Check sheet for the modelled part. Datum: model origin and axes. Units: mm. A direction names the side the tool comes from. Round coordinates to 2 decimals unless told otherwise and drop trailing zeros. Write each loop counter-clockwise with the first axis right and the second up, starting at its lowest first coordinate (ties: lowest second). Pieces come first, ordered by that corner, then holes. Notation, with made-up numbers: (20, 79.5) - (32, 79.5) arc R12 ccw to (32, 92.5) - close; hole circle Ø2 at (-11, -18). An arc over 180 degrees is marked (long way). Use one line per item in the form item = value. Start each with the question number.
1) Section check B-B (y = 20.5). Count the separate pieces of the cut face and the enclosed holes in it, then the cut area to 3 significant figures.
2) Section check D-D (z = 21). Record the boundary of the cut face in (x, y), then the cut area to 3 significant figures.
3) Set-up check for faces 1 (the face through (-13, -25.4, 7)), 2 (the face through (16, 0, -4.762)): record each of +Z, -Z, +X, -X, +Y, -Y from which the full face is reachable in a straight line by a thin tool's end or side.
4) Section check C-C (x = 65). Record the boundary of the cut face in (y, z).
5) Gauge pin test, flat ends, axial feed: P1, Ø3, axis at x = -14.5, y = 7.5, coming from the -Z side; P2, Ø2, axis at y = 20, z = -2, coming from the +X side; P3, Ø6, axis at x = -17, y = 4, coming from the +Z side. Record the tip position at first contact, or that the pin passes through.
6) Draft check along Z on faces 3 (the face through (22, 25.4, 0)), 4 (the face through (30.824, 12.522, -23.504)), 5 (the face through (0.246, 0.356, -14.285)). Enter one of: +Z half, -Z half, draft (parallel to the pull), parting line (faces both ways), or undercut.
7) Section check A-A (x = 0). Record the boundary of the cut face in (y, z) (1 decimal), then the cut area to 3 significant figures.
8) Scan lines: probe 1 along X at (y, z) = (22.5, -0.5); probe 2 along X at (y, z) = (7, 11); probe 3 along Y at (x, z) = (35, 19.5). Record each from-to range of solid material in increasing order.
from build123d import *

# Parameters (mm, degrees)
F0_R     = 14.2875
F1_DEPTH = 25.4
F2_DEPTH = 25.4


with BuildPart() as f1:
    # F0 (on Front) → F1 (new body)
    with BuildSketch(Plane.XZ):
        with BuildLine():
            ThreePointArc((5.042647, -28.126541), (21.916025, -18.336262), (28.575, 0))
            ThreePointArc((28.575, 0), (21.916025, 18.336262), (5.042647, 28.126541))
            ThreePointArc((5.042647, 28.126541), (-28.575, 0), (5.042647, -28.126541))
        make_face()
        with BuildLine():
            ThreePointArc((-13.470384, 4.7625), (0, 14.2875), (13.470384, 4.7625))
            Line((13.470384, 4.7625), (19.05, 4.7625))
            Line((19.05, 4.7625), (19.05, -4.7625))
            Line((19.05, -4.7625), (13.470384, -4.7625))
            ThreePointArc((13.470384, -4.7625), (0, -14.2875), (-13.470384, -4.7625))
            Line((-13.470384, -4.7625), (-19.05, -4.7625))
            Line((-19.05, -4.7625), (-19.05, 4.7625))
            Line((-19.05, 4.7625), (-13.470384, 4.7625))
        make_face(mode=Mode.SUBTRACT)
        with BuildLine():
            ThreePointArc((73.025, 0), (68.585683, 12.224174), (57.336765, 18.751028))
            ThreePointArc((57.336765, 18.751028), (34.925, 0), (57.336765, -18.751028))
            ThreePointArc((57.336765, -18.751028), (68.585683, -12.224174), (73.025, 0))
        make_face()
        with Locations((53.975, 0)):
            Circle(F0_R, mode=Mode.SUBTRACT)
        with BuildLine():
            ThreePointArc((5.042647, 28.126541), (21.916025, 18.336262), (28.575, 0))
            ThreePointArc((28.575, 0), (21.916025, -18.336262), (5.042647, -28.126541))
            Line((5.042647, -28.126541), (57.336765, -18.751028))
            ThreePointArc((57.336765, -18.751028), (34.925, 0), (57.336765, 18.751028))
            Line((57.336765, 18.751028), (5.042647, 28.126541))
        make_face()
    extrude(amount=-F1_DEPTH)

    # F0 (on Front) → F2 (join)
    with BuildSketch(Plane.XZ):
        with BuildLine():
            ThreePointArc((5.042647, -28.126541), (21.916025, -18.336262), (28.575, 0))
            ThreePointArc((28.575, 0), (21.916025, 18.336262), (5.042647, 28.126541))
            ThreePointArc((5.042647, 28.126541), (-28.575, 0), (5.042647, -28.126541))
        make_face()
        with BuildLine():
            ThreePointArc((-13.470384, 4.7625), (0, 14.2875), (13.470384, 4.7625))
            Line((13.470384, 4.7625), (19.05, 4.7625))
            Line((19.05, 4.7625), (19.05, -4.7625))
            Line((19.05, -4.7625), (13.470384, -4.7625))
            ThreePointArc((13.470384, -4.7625), (0, -14.2875), (-13.470384, -4.7625))
            Line((-13.470384, -4.7625), (-19.05, -4.7625))
            Line((-19.05, -4.7625), (-19.05, 4.7625))
            Line((-19.05, 4.7625), (-13.470384, 4.7625))
        make_face(mode=Mode.SUBTRACT)
    extrude(amount=F2_DEPTH)


solid = f1.part
Results are:
q1.separate_pieces = 1
q1.enclosed_holes = 2
q1.area = 3,080 mm²
q2.outline = (-19.38, -25.4) - (19.38, -25.4) - (19.38, 0) - (44.79, 0) - (44.79, 25.4) - (-19.38, 25.4) - close
q2.area = 2,610 mm²
q3.face_1 = +Z, -Z, +X, -X, -Y
q3.face_2 = +Y, -Y
q4.outline = (0, -15.54) - (25.4, -15.54) - (25.4, -9.09) - (0, -9.09) - close; (0, 9.09) - (25.4, 9.09) - (25.4, 15.54) - (0, 15.54) - close
q5.P1 = -25.45
q5.P2 = 73
q5.P3 = 24.91
q6.face_3 = draft
q6.face_4 = -Z half
q6.face_5 = undercut
q7.outline = (-25.4, -28.6) - (25.4, -28.6) - (25.4, -14.3) - (-25.4, -14.3) - close; (-25.4, 14.3) - (25.4, 14.3) - (25.4, 28.6) - (-25.4, 28.6) - close
q7.area = 1,450 mm²
q8.probe_1 = -28.57 to -19.05, 19.05 to 39.7, 68.25 to 73.02
q8.probe_2 = -26.37 to -9.12, 9.12 to 44.86, 63.09 to 69.53
q8.probe_3 = 0 to 25.4
